from build123d import *

# Parameters (mm, degrees)
SKETCH1_W          = 50
SKETCH1_H          = 100
BASE_FLANGE1_DEPTH = 3
EDGE_FLANGE2_DEPTH = 100
SKETCH12_W         = 48.601077025
SKETCH12_H         = 29
CUT_EXTRUDE1_DEPTH = 29
SKETCH13_W         = 48.601077025
SKETCH13_H         = 29
CUT_EXTRUDE2_DEPTH = 29
SKETCH14_W         = 80
SKETCH14_H         = 20
TAB1_DEPTH         = 3


# Sheet-metal steps are written as plain solids
with BuildPart() as part:
    # Sketch1 → Base-Flange1 (new body)
    with BuildSketch(Plane.XY):
        with Locations((-11.571125265, -23.036093418)):
            Rectangle(SKETCH1_W, SKETCH1_H)
    extrude(amount=-BASE_FLANGE1_DEPTH)

    # Edge-Flange2 section (across the edge) → Edge-Flange2 (add)
    with BuildSketch(Plane(origin=(14.827797709, -73.036093418, 0), x_dir=(-0.7660444431189746, 0, 0.6427876096865435), z_dir=(0, 1, 0))):
        with BuildLine():
            Line((-3, 1.398922974), (-3, 50))
            Line((-3, 50), (0, 50))
            Line((0, 50), (0, 1.398922974))
            ThreePointArc((0, 1.398922974), (0.281076639, 0.131068189), (1.071637171, -0.899210355))
            Line((1.071637171, -0.899210355), (-0.856725658, -3.197343684))
            ThreePointArc((-0.856725658, -3.197343684), (-2.437846722, -1.136786596), (-3, 1.398922974))
        make_face()
    extrude(amount=EDGE_FLANGE2_DEPTH)

    # Sketch12 → Cut-Extrude1 (cut)
    with BuildSketch(Plane(origin=(8.70130888, 0, -7.301265072), x_dir=(0.6427876096865439, 0, 0.7660444431189742), z_dir=(-0.7660444431189742, 0, 0.6427876096865439))):
        with Locations((35.230586133, -1.536093418)):
            Rectangle(SKETCH12_W, SKETCH12_H)
    extrude(amount=-CUT_EXTRUDE1_DEPTH, mode=Mode.SUBTRACT)

    # Sketch13 → Cut-Extrude2 (cut)
    with BuildSketch(Plane(origin=(8.70130888, 0, -7.301265072), x_dir=(0.6427876096865439, 0, 0.7660444431189742), z_dir=(-0.7660444431189742, 0, 0.6427876096865439))):
        with Locations((35.230586133, -44.536093418)):
            Rectangle(SKETCH13_W, SKETCH13_H)
    extrude(amount=-CUT_EXTRUDE2_DEPTH, mode=Mode.SUBTRACT)

    # Sketch14 → Tab1 (add)
    with BuildSketch(Plane.XY):
        with Locations((-36.571125265, -23.036093418)):
            Rectangle(SKETCH14_W, SKETCH14_H)
    extrude(amount=-TAB1_DEPTH)


solid = part.part
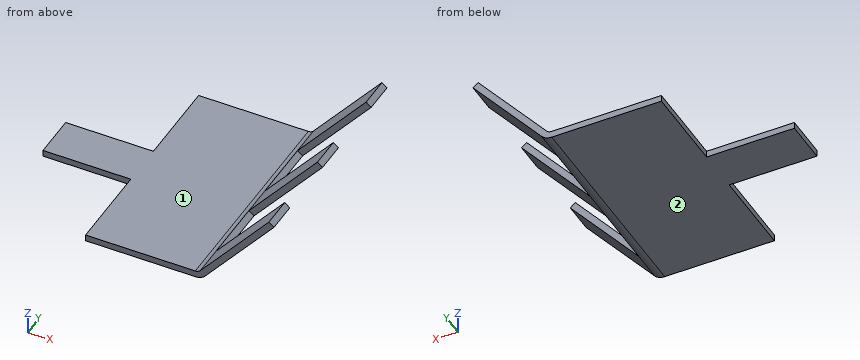
Can you work these out from the model? Positions are in its coordinate system, mm. Face numbers are marked on the shaded views. A direction names the side the tool comes from. Coordinates: 2 decimals unless noted, no trailing zeros. Write each loop counter-clockwise with the first axis right and the second up, starting at its lowest first coordinate (ties: lowest second). Pieces come first, ordered by that corner, then holes. Notation, with made-up numbers: (72, -29.5) -> (88, -29.5) arc R21 ccw to (88, -10.5) -> close; hole circle Ø7 at (46, 32.5). An arc over 180 degrees is marked (long way). Answer as CSV lines item,"result".
1) If we section it at A-A on z = 29: Please give me the cut outline in (x, y), then the cut area to 3 significant figures.
Check result:
outline,"(39.16, -73.04) -> (43.08, -73.04) -> (43.08, -59.04) -> (39.16, -59.04) -> close; (39.16, -30.04) -> (43.08, -30.04) -> (43.08, -16.04) -> (39.16, -16.04) -> close; (39.16, 12.96) -> (43.08, 12.96) -> (43.08, 26.96) -> (39.16, 26.96) -> close"
area,"164 mm²"
2) On a 3-axis mill with a long thin cutter (end or side, diameter ignored), from which of +Z, -Z, +X, -X, +Y, -Y can I reach the whole of each face in a straight line? I mean the marked faces 1 and 2. Say none if no direction works.
Check result:
face 1,"+Z, -X, +Y, -Y"
face 2,"-Z, +X, -X, +Y, -Y"
3) Will these pins go through, and if not, where does the flat tip stop? P1, Ø0.9, axis at y = -47, z = -2, coming from the -X side; P2, Ø3.5, axis at x = -53.5, z = -2, coming from the +Y side; P3, Ø3.5, axis at x = -58.5, z = -1.5, coming from the -Y side.
Check result:
P1,"x = -36.57"
P2,"y = -13.04"
P3,"y = -33.04"
4) If we section it at C-C on x = -51: Please give me the cut outline in (y, z).
Check result:
outline,"(-33.04, -3) -> (-13.04, -3) -> (-13.04, 0) -> (-33.04, 0) -> close"
5) If we section it at D-D on y = -41.5: Please give me the cut outline in (x, z), then the cut area to 3 significant figures.
Check result:
outline,"(-36.57, -3) -> (13.43, -3) arc R6 ccw to (18.03, -0.86) -> (15.73, 1.07) arc R3 cw to (13.43, 0) -> (-36.57, 0) -> close"
area,"162 mm²"
6) If we section it at B-B on y = 20: Please give me the cut outline in (x, z), then the cut area to 3 significant figures.
Check result:
outline,"(-36.57, -3) -> (13.43, -3) arc R6 ccw to (18.03, -0.86) -> (49.27, 36.37) -> (46.97, 38.3) -> (15.73, 1.07) arc R3 cw to (13.43, 0) -> (-36.57, 0) -> close"
area,"308 mm²"
7) If I drill on line 1 (Y direction, x = 38.5, z = 27); line 2 (Z direction, x = -63.5, y = -28); line 3 (Y direction, x = -55, z = -0.5), over which ranges is the centre line in solid material (lowest first)? Write a range as from..to.
Check result:
line 1,"-73.04..-59.04, -30.04..-16.04, 12.96..26.96"
line 2,"-3..0"
line 3,"-33.04..-13.04"
